For this review, take the finished solid that the model builds, in its own axes (mm). Face numbers are marked on the shaded views. A direction names the side the tool comes from. Round coordinates to 2 decimals unless told otherwise and drop trailing zeros. Write each loop counter-clockwise with the first axis right and the second up, starting at its lowest first coordinate (ties: lowest second). Pieces come first, ordered by that corner, then holes. Notation, with made-up numbers: (-30.75, 37) -> (-15.75, 37) arc R24 cw to (-15.75, 76) -> close; hole circle Ø3 at (7, 53.5). An arc over 180 degrees is marked (long way). Answer as CSV lines item,"result". Start each with the question number.
Item 1: Machinability: for the marked faces 4 and 5, which of the approach directions +Z, -Z, +X, -X, +Y, -Y give a long, thin tool a straight path to every point of the face, cutting with its end or side? Answer none if there is none.
Item 2: Take a section at B-B on z = 15.5. Give the boundary of the cut face in (x, y).
Item 3: Mouldability with a two-part tool opening along Y and no side actions: class the marked faces 1, 2 and 3 as +Y half, -Y half, draft (parallel to the pull), parting line (faces both ways), or undercut.
Item 4: Take a section at A-A on y = -23.5. Give the boundary of the cut face in (x, z).
Item 5: Wall thickness on probe 1 along X at (y, z) = (-24.5, 2.25); probe 2 along Y at (x, z) = (3, 5.5); probe 3 along Z at (x, y) = (14.5, -22.5): over which ranges is each line inside the solid? List them lowest first. Write a range as from..to.
Item 6: Take a section at D-D on x = 8.75. Give the boundary of the cut face in (y, z), then the cut area to 3 significant figures.
Item 7: For pin 1 Ø1 at (x, y) = (10.5, -25) entering from +Z, flat-tipped, find the tip position at first contact; note if it passes through.
Item 8: Take a section at C-C on x = 12.5. Give the boundary of the cut face in (y, z).
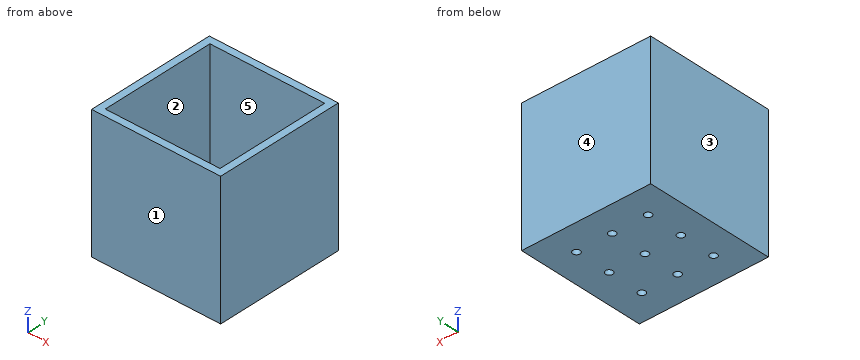
```python
from build123d import *

# Parameters (mm, degrees)
F0_W     = 18
F0_H     = 18
F1_DEPTH = 18.5
F2_T     = -1
F4_D     = 1


with BuildPart() as f1:
    # F0 (on Top) → F1 (new body)
    with BuildSketch(Plane.XY):
        with Locations((7.472297, -17.565783)):
            Rectangle(F0_W, F0_H)
    extrude(amount=F1_DEPTH)

    # F2
    f2_openings = [f1.faces().sort_by_distance(p)[0] for p in [
        (7.472297, -17.565783, 18.5),
    ]]
    offset(amount=F2_T, openings=f2_openings)

    # F4 (through all)
    with Locations(Plane(origin=(0, 0, 0), x_dir=(1, 0, 0), z_dir=(0, 0, -1))):
        with Locations((12.472297, 22.565783), (7.472297, 17.565783), (2.472297, 12.565783), (7.472297, 12.565783), (12.472297, 12.565783), (12.472297, 17.565783), (2.472297, 17.565783), (2.472297, 22.565783), (7.472297, 22.565783)):
            Hole(F4_D / 2)


solid = f1.part
```
Output values:
1,face 4,"+Z, -Z, +X, -X, +Y"
1,face 5,"+Z"
2,outline,"(-1.53, -26.57) -> (16.47, -26.57) -> (16.47, -8.57) -> (-1.53, -8.57) -> close; hole (-0.53, -25.57) -> (15.47, -25.57) -> (15.47, -9.57) -> (-0.53, -9.57) -> close"
3,face 1,"-Y half"
3,face 2,"undercut"
3,face 3,"draft"
4,outline,"(-1.53, 0) -> (16.47, 0) -> (16.47, 18.5) -> (15.47, 18.5) -> (15.47, 1) -> (-0.53, 1) -> (-0.53, 18.5) -> (-1.53, 18.5) -> close"
5,probe 1,"x = -1.53..-0.53, 15.47..16.47"
5,probe 2,"y = -26.57..-25.57, -9.57..-8.57"
5,probe 3,"z = 0..1"
6,outline,"(-26.57, 0) -> (-8.57, 0) -> (-8.57, 18.5) -> (-9.57, 18.5) -> (-9.57, 1) -> (-25.57, 1) -> (-25.57, 18.5) -> (-26.57, 18.5) -> close"
6,area,"53.0 mm^2"
7,pin 1,"stops at z = 1"
8,outline,"(-26.57, 0) -> (-23.07, 0) -> (-23.07, 1) -> (-25.57, 1) -> (-25.57, 18.5) -> (-26.57, 18.5) -> close; (-22.07, 0) -> (-18.07, 0) -> (-18.07, 1) -> (-22.07, 1) -> close; (-17.07, 0) -> (-13.07, 0) -> (-13.07, 1) -> (-17.07, 1) -> close; (-12.07, 0) -> (-8.57, 0) -> (-8.57, 18.5) -> (-9.57, 18.5) -> (-9.57, 1) -> (-12.07, 1) -> close"
